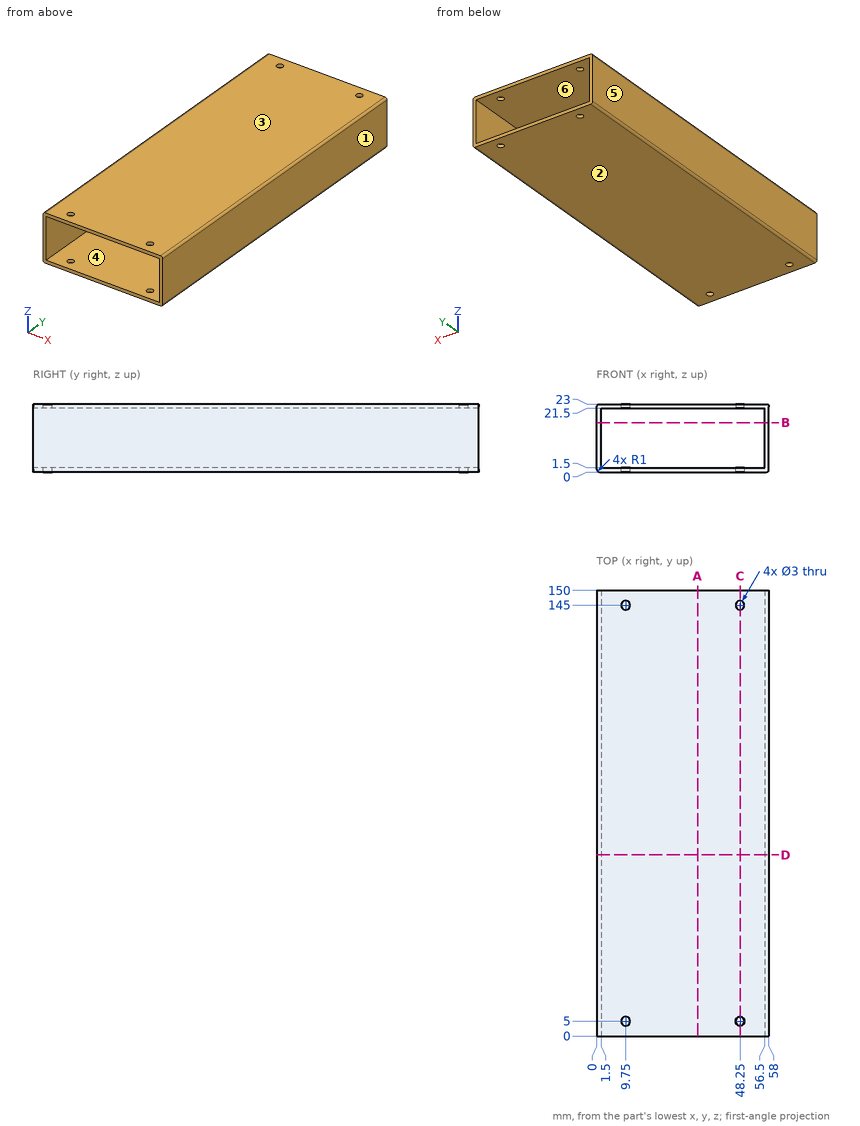
Check sheet for the drawn part. Datum: minimum x, y, z corner. Units: mm. A direction names the side the tool comes from. Round coordinates to 2 decimals unless told otherwise and drop trailing zeros. Loops run counter-clockwise (first coordinate to the right, second up) from the corner with the lowest first, then second, coordinate; pieces in that order, holes last. Notation, with made-up numbers: (81, -16.75) - (104, -16.75) arc R20 ccw to (104, -9.75) - close; hole circle Ø1 at (78, -34.5). An arc over 180 degrees is marked (long way). Answer as a JSON object with one key per item and string values. Group by question number.
Q1. Sectioned sample at B-B, the plane z = 16.75. Enter the section's corners in (x, y), plus the area to 3 significant figures.
Q2. Set-up check for the marked faces 5 and 6: record each of +Z, -Z, +X, -X, +Y, -Y from which the full face is reachable in a straight line by a thin tool's end or side.
Q3. Gauge pin test, flat ends, axial feed: P1, Ø12, axis at y = 126.5, z = 17.5, coming from the -X side; P2, Ø8, axis at x = 24.5, z = 8, coming from the +Y side. Record the tip position at first contact, or that the pin passes through.
Q4. Mould release check, pull along Z, two halves, no side actions. Record for the marked faces 1, 2, 3 and 4: released by +Z, released by -Z, zero draft, split by the parting line, or undercut.
Q5. Sectioned sample at D-D, the plane y = 61. Enter the section's corners in (x, z), plus the area to 3 significant figures.
Q6. Sectioned sample at C-C, the plane x = 48.25. Enter the section's corners in (y, z), plus the area to 3 significant figures.
Q7. Sectioned sample at A-A, the plane x = 34. Enter the section's corners in (y, z), plus the area to 3 significant figures.
Q8. Scan lines: line 1 along Y through (x, z) = (9.75, 0.65); line 2 along X through (y, z) = (145, 22.25); line 3 along X through (y, z) = (135.5, 12). Record each from-to range of solid material in increasing order. Write a range as [from, to].
Solution:
{
 "1": {"outline": "(0, 0) - (1.5, 0) - (1.5, 150) - (0, 150) - close; (56.5, 0) - (58, 0) - (58, 150) - (56.5, 150) - close", "area": "450 mm²"},
 "2": {"face 5": "+Z, -Z, -X, +Y, -Y", "face 6": "+Y, -Y"},
 "3": {"P1": "stops at x = 0", "P2": "passes through"},
 "4": {"face 1": "zero draft", "face 2": "released by -Z", "face 3": "released by +Z", "face 4": "undercut"},
 "5": {"outline": "(0, 1) arc R1 ccw to (1, 0) - (57, 0) arc R1 ccw to (58, 1) - (58, 22) arc R1 ccw to (57, 23) - (1, 23) arc R1 ccw to (0, 22) - close; hole (1.5, 1.5) - (56.5, 1.5) - (56.5, 21.5) - (1.5, 21.5) - close", "area": "233 mm²"},
 "6": {"outline": "(0, 0) - (3.5, 0) - (3.5, 1.5) - (0, 1.5) - close; (0, 21.5) - (3.5, 21.5) - (3.5, 23) - (0, 23) - close; (6.5, 0) - (143.5, 0) - (143.5, 1.5) - (6.5, 1.5) - close; (6.5, 21.5) - (143.5, 21.5) - (143.5, 23) - (6.5, 23) - close; (146.5, 0) - (150, 0) - (150, 1.5) - (146.5, 1.5) - close; (146.5, 21.5) - (150, 21.5) - (150, 23) - (146.5, 23) - close", "area": "432 mm²"},
 "7": {"outline": "(0, 0) - (150, 0) - (150, 1.5) - (0, 1.5) - close; (0, 21.5) - (150, 21.5) - (150, 23) - (0, 23) - close", "area": "450 mm²"},
 "8": {"line 1": "y = [0, 3.5], [6.5, 143.5], [146.5, 150]", "line 2": "x = [0.03, 8.25], [11.25, 46.75], [49.75, 57.97]", "line 3": "x = [0, 1.5], [56.5, 58]"}
}
